from build123d import *

# Parameters (mm, degrees)
SKETCH7_R            = 22
SKETCH7_R_2          = 20
BOSS_EXTRUDE7_DEPTH  = 5
SKETCH8_R            = 8
SKETCH8_R_2          = 5
BOSS_EXTRUDE8_DEPTH  = 13
BOSS_EXTRUDE10_DEPTH = 3
CIRPATTERN2_COUNT    = 3


with BuildPart() as part:
    # Sketch7 → Boss-Extrude7 (new body)
    with BuildSketch(Plane.XY):
        Circle(SKETCH7_R)
        Circle(SKETCH7_R_2, mode=Mode.SUBTRACT)
    extrude(amount=BOSS_EXTRUDE7_DEPTH)



with BuildPart() as body_2:
    # Sketch8 → Boss-Extrude8 (new body)
    with BuildSketch(Plane.XY):
        Circle(SKETCH8_R)
        Circle(SKETCH8_R_2, mode=Mode.SUBTRACT)
    extrude(amount=BOSS_EXTRUDE8_DEPTH)


with BuildPart() as part_1:
    add(part.part)

    add(body_2.part)  # Boss-Extrude10 merges body 2
    # Sketch9 → Boss-Extrude10 (add)
    with BuildSketch(Plane(origin=(0, 0, 0), x_dir=(0, 0, -1), z_dir=(1, 0, 0))):
        Polygon((-13, 8), (-5, 20), (0, 20), (0, 8), (0, 5), (-13, 5), align=None)
    boss_extrude10 = extrude(amount=BOSS_EXTRUDE10_DEPTH)

    # CirPattern2: Boss-Extrude10 ×3 about axis
    cirpattern2_axis = Axis((0, 0, 0), (0, 0, 1))
    for i in range(1, CIRPATTERN2_COUNT):
        add(boss_extrude10.rotate(cirpattern2_axis, i * 360 / CIRPATTERN2_COUNT))


solid = part_1.part
Read the model definition and answer for the solid it produces. Units are mm, in the model's axes. A direction names the side the tool comes from. Coordinates: 2 decimals unless noted, no trailing zeros. Write each loop counter-clockwise with the first axis right and the second up, starting at its lowest first coordinate (ties: lowest second). Pieces come first, ordered by that corner, then holes. Notation, with made-up numbers: M 47,-22 L 63,-22 A12 ccw 63,-9 Z; hole C 86.5,86.5 d11. An arc over 180 degrees is marked long. Use a Markdown table: item, result.
Q1. The part is cut by section C-C, the plane z = 12. Write down the section's boundary in (x, y).
Answer block:
| item | result |
|---|---|
| outline | M -9.73,-2.15 L -8.23,-4.75 L -6.93,-4 A8 ccw 4.92,-6.31 L 6.73,-7.35 L 8.23,-4.75 L 6.93,-4 A8 ccw 3,7.42 L 3,9.5 L 0,9.5 L 0,8 A8 ccw -7.92,-1.11 Z; hole C 0,0 d10 |
Q2. Each of these flat-tipped pins is pushed along its axis until it touches: pin 1 Ø1.5 at (x, z) = (11.5, 9.5) entering from +Y; pin 2 Ø6 at (y, z) = (12, 9) entering from -X; pin 3 Ø13 at (x, y) = (-8, -4.5) entering from +Z; pin 4 Ø4 at (y, z) = (12, 9) entering from +X. Where does it stop, or does it pass through?
Answer block:
| item | result |
|---|---|
| pin 1 | stops at y = -6.21 |
| pin 2 | stops at x = 0 |
| pin 3 | stops at z = 13 |
| pin 4 | stops at x = 3 |
Q3. Which of the six approach directions +Z, -Z, +X, -X, +Y, -Y give full straight-line access (tool end or side, diameter ignored) to faces 5 (the face through (-5.1, 1.2, 0)), 6 (the face through (11.042, -6.375, 4.965))?
Answer block:
| item | result |
|---|---|
| face 5 | -Z, +X, -X, +Y, -Y |
| face 6 | +Z, -Z |
Q4. Determine the mould class of faces 1 (the face through (18.14, 8.42, 2.46)), 2 (the face through (-1.78, -19.92, 2.46)), 3 (the face through (11.312, -8.239, 9.056)), 4 (the face through (10, -18, 5)) for opening direction X: released by +X, released by -X, zero draft, split by the parting line, or undercut.
Answer block:
| item | result |
|---|---|
| face 1 | undercut |
| face 2 | undercut |
| face 3 | released by +X |
| face 4 | zero draft |
Q5. The part is cut by section D-D, the plane x = -3. Write down the section's boundary in (y, z), then the cut area to 3 significant figures.
Answer block:
| item | result |
|---|---|
| outline | M -21.79,0 L -19.77,0 L -19.77,5 L -21.79,5 Z; M -7.42,0 L -4,0 L -4,13 L -7.42,13 Z; M 4,0 L 7.42,0 L 7.42,13 L 4,13 Z; M 19.77,0 L 21.79,0 L 21.79,5 L 19.77,5 Z |
| area | 109 mm2 |
Q6. Straight lines are drawn through the part: L1, parallel to X at y = 0, z = 10; L2, parallel to Y at x = -2, z = 1; L3, parallel to Y at x = -13.5, z = 2.5. For each, find the intervals that lie inside material, in ascending order. Write a range as [from, to].
Answer block:
| item | result |
|---|---|
| L1 | x = [-8, -5], [5, 8] |
| L2 | y = [-21.91, -19.9], [-7.75, -4.58], [4.58, 7.75], [19.9, 21.91] |
| L3 | y = [-17.37, -14.76], [-7.79, -4.33], [14.76, 17.37] |
Q7. The part is cut by section A-A, the plane y = 0. Write down the section's boundary in (x, z).
Answer block:
| item | result |
|---|---|
| outline | M -22,0 L -20,0 L -20,5 L -22,5 Z; M -8,0 L -5,0 L -5,13 L -8,13 Z; M 5,0 L 8,0 L 8,13 L 5,13 Z; M 20,0 L 22,0 L 22,5 L 20,5 Z |
Q8. The part is cut by section B-B, the plane x = 1.5. Write down the section's boundary in (y, z).
Answer block:
| item | result |
|---|---|
| outline | M -21.95,0 L -19.94,0 L -19.94,5 L -21.95,5 Z; M -7.86,0 L -4.77,0 L -4.77,13 L -7.86,13 Z; M 4.77,0 L 21.95,0 L 21.95,5 L 20,5 L 8,13 L 4.77,13 Z |
